Geometry: final body of the model. Coordinates: model frame, mm. A direction names the side the tool comes from. Give positions to 0.01 mm unless a question says otherwise; leave off trailing zeros. Write each loop counter-clockwise with the first axis right and the second up, starting at its lowest first coordinate (ties: lowest second). Pieces come first, ordered by that corner, then holes. Notation, with made-up numbers: (65, 63) -> (78, 63) arc R5 cw to (78, 72) -> close; hole circle Ø10 at (-30, 62.5). An arc over 180 degrees is marked (long way). Answer as a JSON object with one key per item and string values.
from build123d import *

# Parameters (mm, degrees)
PAD_DEPTH     = 1.65
SKETCH001_R   = 2.195453
SKETCH001_R_2 = 8.192022
SKETCH001_R_3 = 5.613861
SKETCH001_R_4 = 14.865337
SKETCH001_R_5 = 10.448492
PAD001_DEPTH  = 3.15
SKETCH002_W   = 13.5
SKETCH002_H   = 13
PAD002_DEPTH  = 9.6


with BuildPart() as part:
    # Sketch → Pad (new body)
    with BuildSketch(Plane.XY):
        Polygon((-110.5, 50), (80, 50), (80, -55.8), (64.15, -55.8), (64.15, -46.55), (34.45, -46.55), (34.45, -61.1), (-50.55, -61.1), (-50.55, -48), (-110.5, -48), align=None)
    extrude(amount=PAD_DEPTH)

    # Sketch001 (on Face12 of Pad) → Pad001 (join)
    with BuildSketch(Plane.XY.offset(1.65)):
        with Locations((-43.015316, 33.133453)):
            Circle(SKETCH001_R)
        with Locations((22.746756, 31.915638)):
            Circle(SKETCH001_R_2)
        with Locations((-67.77758, -4.618844)):
            Circle(SKETCH001_R_3)
        with Locations((25.994263, -10.707931)):
            Circle(SKETCH001_R_4)
        with Locations((-23.936199, -16.188095)):
            Circle(SKETCH001_R_5)
    extrude(amount=PAD001_DEPTH)

    # Sketch002 (on Face4 of Pad001) → Pad002 (join)
    with BuildSketch(Plane(origin=(0, 0, 0), x_dir=(1, 0, 0), z_dir=(0, 0, -1))):
        with Locations((-102.75, -43.5)):
            Rectangle(SKETCH002_W, SKETCH002_H)
    extrude(amount=PAD002_DEPTH)


solid = part.part
Q1. Material intervals for L1, parallel to X at y = -49.5, z = 1.5; L2, parallel to Z at x = 39, y = 9.5; L3, parallel to X at y = -11.5, z = 2.5, sorted ascending. Write a range as from..to.
Values:
{"L1": "-50.55..34.45, 64.15..80", "L2": "0..1.65", "L3": "-33.27..-14.6, 11.15..40.84"}
Q2. Cut plane C-C (z = -5.75). Return the cut outline in (x, y), and give its area (4 significant figures).
Values:
{"outline": "(-109.5, 37) -> (-96, 37) -> (-96, 50) -> (-109.5, 50) -> close", "area": "175.5 mm²"}
Q3. Cut plane A-A (y = -20). Return the cut outline in (x, z), and give its area (3 significant figures).
Values:
{"outline": "(-110.5, 0) -> (80, 0) -> (80, 1.65) -> (37.6, 1.65) -> (37.6, 4.8) -> (14.39, 4.8) -> (14.39, 1.65) -> (-14.21, 1.65) -> (-14.21, 4.8) -> (-33.66, 4.8) -> (-33.66, 1.65) -> (-110.5, 1.65) -> close", "area": "449 mm²"}
Q4. Mould query, pull axis X, two halves, no side actions, for faces 4 (the cylindrical face through (-31.64, -9.13, 3.2)), 5 (the flat face through (-109.5, 44, -5)), 6 (the flat face through (23, 32, 4.8)). Classes: pulls with the +X half, pulls with the -X half, needs draft (parallel to the pull), parting line crosses it, or undercut.
Values:
{"face 4": "undercut", "face 5": "pulls with the -X half", "face 6": "needs draft"}
Q5. Cut plane D-D (x = 24). Return the cut outline in (y, z), and give its area (3 significant figures).
Values:
{"outline": "(-61.1, 0) -> (50, 0) -> (50, 1.65) -> (40.01, 1.65) -> (40.01, 4.8) -> (23.82, 4.8) -> (23.82, 1.65) -> (4.02, 1.65) -> (4.02, 4.8) -> (-25.44, 4.8) -> (-25.44, 1.65) -> (-61.1, 1.65) -> close", "area": "327 mm²"}
Q6. Set-up query: faces 1 (the cylindrical face through (-73.386, -4.372, 3.203)), 2 (the flat face through (-96, 44, -5)), 3 (the flat face through (-103, 37, -5)). Return all of +Z, -Z, +X, -X, +Y, -Y with unobstructed straight access to the full face (end or side cutting, diameter ignored); none if empty.
Values:
{"face 1": "+Z", "face 2": "-Z, +X, +Y, -Y", "face 3": "-Z, +X, -X, -Y"}
Q7. Cut plane B-B (x = -83.5). Return the cut outline in (y, z), and give its area (3 significant figures).
Values:
{"outline": "(-48, 0) -> (50, 0) -> (50, 1.65) -> (-48, 1.65) -> close", "area": "162 mm²"}
Q8. First-contact query: P1, Ø6, axis at x = 23, z = -4.5, coming from the +Y side; P2, Ø1.8, axis at x = 50, z = 1, coming from the -Y side; P3, Ø2, axis at x = 23.5, y = 29, coming from the -Z side; P4, Ø2, axis at x = 39, y = 15.5, coming from the +Z side. Flat tips, straight axial feed; report the tip coordinate or a pass-through.
Values:
{"P1": "through", "P2": "y = -46.55", "P3": "z = 0", "P4": "z = 1.65"}
